Drawing for the job (mm, zero at the part's lowest x, y, z). A direction names the side the tool comes from. Coordinates: 2 decimals unless noted, no trailing zeros. Order: outer loops, then holes, each group sorted by start corner. A loop starts at its lowest first (then second) coordinate and runs counter-clockwise, first axis right, second up.
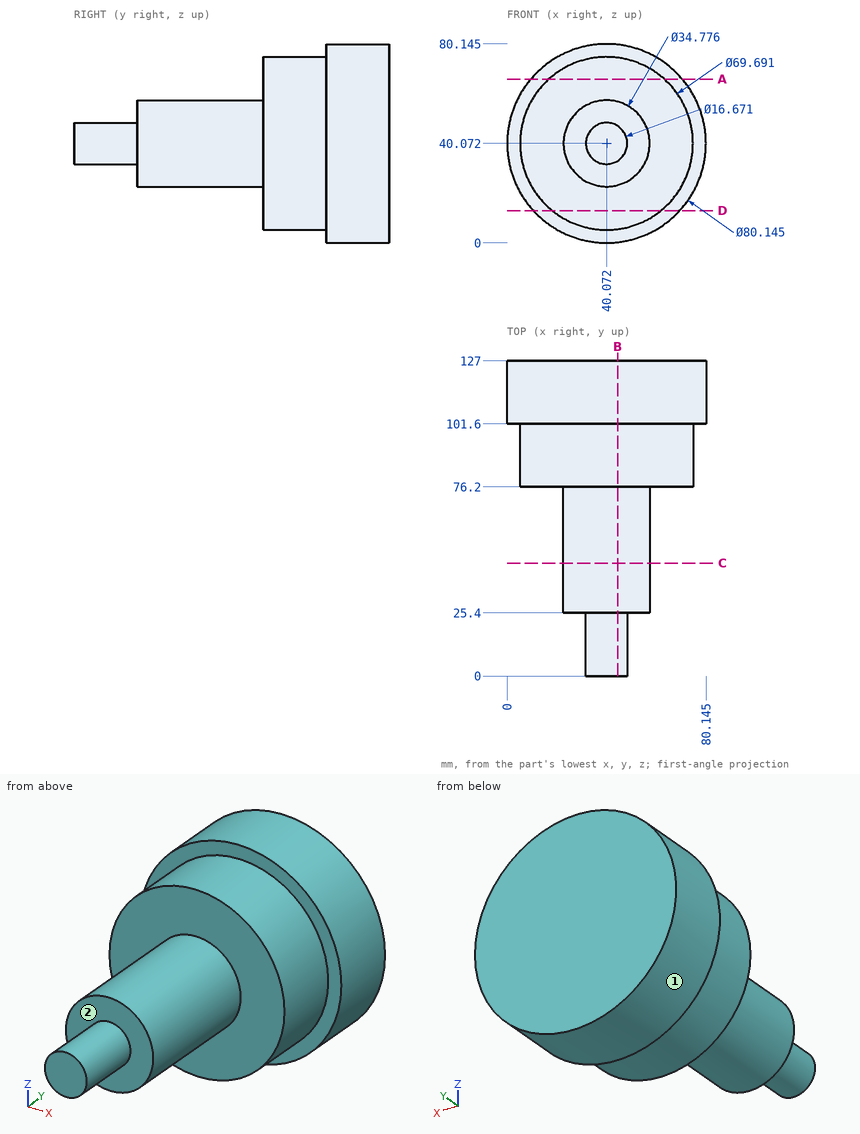
(1) Slice it at B-B, the plane x = 44.5. Give the cut face in (y, z) (1 decimal).
(2) Slice it at A-A, the plane z = 66. Give the cut face in (x, y), then the cut area to 3 significant figures.
(3) Probe line 1 (Y direction, x = 70.5, z = 43.5); line 2 (Y direction, x = 45, z = 56); line 3 (X direction, y = 118, z = 45) (1 decimal). List the from-to ranges inside material, lowest first.
(4) Slice it at C-C, the plane y = 45.5. Give the cut face in (x, z) (1 decimal).
(5) Tool access for the marked faces 1 and 2: list every direction of +Z, -Z, +X, -X, +Y, -Y with a clear straight run to the whole face (end or side of a thin tool).
(6) Slice it at D-D, the plane z = 13. Give the cut face in (x, y), then the cut area to 3 significant figures.
(7) Drop flat-ended pins along their axis: pin 1 (2 mm diameter, centred on x = 18, z = 34.5, fed in from -Y); pin 2 (12 mm diameter, centred on x = 59, y = 110, fed in from -Z); pin 3 (8 mm diameter, centred on y = 84.5, z = 35, fed in from -X); pin 4 (12 mm diameter, centred on x = 69, y = 32, fed in from +Z). Give the stop position or say it passes through.
Here are the results:
1. outline: (0, 33) - (25.4, 33) - (25.4, 23.3) - (76.2, 23.3) - (76.2, 5.5) - (101.6, 5.5) - (101.6, 0.2) - (127, 0.2) - (127, 79.9) - (101.6, 79.9) - (101.6, 74.6) - (76.2, 74.6) - (76.2, 56.9) - (25.4, 56.9) - (25.4, 47.1) - (0, 47.1) - close
2. outline: (9.52, 101.6) - (16.79, 101.6) - (16.79, 76.2) - (63.35, 76.2) - (63.35, 101.6) - (70.63, 101.6) - (70.63, 127) - (9.52, 127) - close
2. area: 2,730 mm2
3. line 1: y = 76.2 to 127
3. line 2: y = 25.4 to 127
3. line 3: x = 0.3 to 79.8
4. outline: circle Ø34.8 at (40.1, 40.1)
5. face 1: +Y, -Y
5. face 2: -Y
6. outline: (10.53, 101.6) - (18.13, 101.6) - (18.13, 76.2) - (62.01, 76.2) - (62.01, 101.6) - (69.62, 101.6) - (69.62, 127) - (10.53, 127) - close
6. area: 2,620 mm2
7. pin 1: stops at y = 76.2
7. pin 2: stops at z = 2.14
7. pin 3: stops at x = 5.24
7. pin 4: passes through
